For this review, take the finished solid that the model builds, in its own axes (mm). Face numbers are marked on the shaded views. A direction names the side the tool comes from. Round coordinates to 2 decimals unless told otherwise and drop trailing zeros. Write each loop counter-clockwise with the first axis right and the second up, starting at its lowest first coordinate (ties: lowest second). Pieces come first, ordered by that corner, then holes. Notation, with made-up numbers: M 79,-36 L 128,-36 A13 ccw 128,-28 Z; hole C -6.5,32 d1. An arc over 180 degrees is marked long. Write each question's results on one line, items separated by ' | '. Start each with the question number.
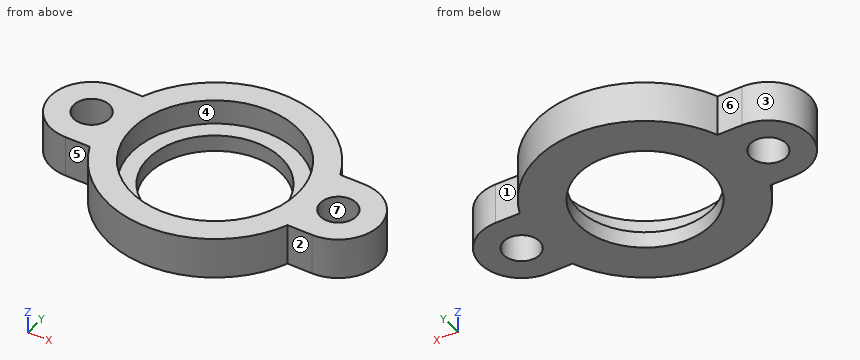
```python
from build123d import *

# Parameters (mm, degrees)
F0_R     = 1.7272
F0_R_2   = 6.4135
F1_DEPTH = 1.5875
F2_R     = 1.7272
F2_R_2   = 8.001
F3_DEPTH = 2.396515


with BuildPart() as f1:
    # F0 (on Top) → F1 (new body)
    with BuildSketch(Plane.XY):
        with BuildLine():
            Line((2.375995, 3.96875), (0, 3.96875))
            ThreePointArc((0, 3.96875), (-3.96875, 0), (0, -3.96875))
            Line((0, -3.96875), (2.375995, -3.96875))
            ThreePointArc((2.375995, -3.96875), (11.96975, -10.38225), (21.563505, -3.96875))
            Line((21.563505, -3.96875), (23.9395, -3.96875))
            ThreePointArc((23.9395, -3.96875), (27.90825, 0), (23.9395, 3.96875))
            Line((23.9395, 3.96875), (21.563505, 3.96875))
            ThreePointArc((21.563505, 3.96875), (11.96975, 10.38225), (2.375995, 3.96875))
        make_face()
        Circle(F0_R, mode=Mode.SUBTRACT)
        with Locations((11.96975, 0)):
            Circle(F0_R_2, mode=Mode.SUBTRACT)
        with Locations((23.9395, 0)):
            Circle(F0_R, mode=Mode.SUBTRACT)
    extrude(amount=F1_DEPTH)

    # F2 (on face) → F3 (join)
    with BuildSketch(Plane.XY.offset(1.5875)):
        with BuildLine():
            Line((23.9395, 3.96875), (21.563505, 3.96875))
            ThreePointArc((21.563505, 3.96875), (11.96975, 10.38225), (2.375995, 3.96875))
            Line((2.375995, 3.96875), (0, 3.96875))
            ThreePointArc((0, 3.96875), (-3.96875, 0), (0, -3.96875))
            Line((0, -3.96875), (2.375995, -3.96875))
            ThreePointArc((2.375995, -3.96875), (11.96975, -10.38225), (21.563505, -3.96875))
            Line((21.563505, -3.96875), (23.9395, -3.96875))
            ThreePointArc((23.9395, -3.96875), (27.90825, 0), (23.9395, 3.96875))
        make_face()
        Circle(F2_R, mode=Mode.SUBTRACT)
        with Locations((11.96975, 0)):
            Circle(F2_R_2, mode=Mode.SUBTRACT)
        with Locations((23.9395, 0)):
            Circle(F2_R, mode=Mode.SUBTRACT)
    extrude(amount=F3_DEPTH)


solid = f1.part
```
Item 1: Mouldability with a two-part tool opening along Y and no side actions: class the marked faces 5, 6 and 7 as pulls with the +Y half, pulls with the -Y half, needs draft (parallel to the pull), parting line crosses it, or undercut.
Item 2: We need section D-D on y = 5.75. State the section outline as (x, z) points, then the cut area to 3 significant figures.
Item 3: For probe 1 along Y at (x, z) = (0, 2.25); probe 2 along X at (y, z) = (-0.75, 3.4); probe 3 along Y at (x, z) = (10.5, 1.55), list the stretches that pass through material, from the lowest coordinate up.
Item 4: We need section B-B on y = 0. State the section outline as (x, z) points, then the cut area to 3 significant figures.
Item 5: We need section A-A on z = 2.9. State the section outline as (x, y) points.
Item 6: For the marked faces 1, 2, 3 and 4, list the 3-axis set-ups (+Z, -Z, +X, -X, +Y, -Y) from which the entire face can be reached by the end or side of a thin tool; tool diameter is ignored.
Item 7: We need section C-C on x = 11. State the section outline as (y, z) points.
Item 8: Insertion check: P1, Ø1, axis at x = 22, z = 3, coming from the -Y side; P2, Ø0.7, axis at x = 23.5, z = 1.5, coming from the -Y side; P3, Ø1, axis at x = 4, z = 2, coming from the +Y side. Each pin has a flat end and moves straight along its axis. Give the tip position at first contact, or say it passes through.
Numbers:
1) face 5: pulls with the -Y half | face 6: pulls with the +Y half | face 7: undercut
2) outline: M 3.33,0 L 9.13,0 L 9.13,1.59 L 6.41,1.59 L 6.41,3.98 L 3.33,3.98 Z; M 14.81,0 L 20.61,0 L 20.61,3.98 L 17.53,3.98 L 17.53,1.59 L 14.81,1.59 Z | area: 33.2 mm^2
3) probe 1: y = -3.97 to -1.73, 1.73 to 3.97 | probe 2: x = -3.9 to -1.56, 1.56 to 4, 19.94 to 22.38, 25.5 to 27.84 | probe 3: y = -10.28 to -6.24, 6.24 to 10.28
4) outline: M -3.97,0 L -1.73,0 L -1.73,3.98 L -3.97,3.98 Z; M 1.73,0 L 5.56,0 L 5.56,1.59 L 3.97,1.59 L 3.97,3.98 L 1.73,3.98 Z; M 18.38,0 L 22.21,0 L 22.21,3.98 L 19.97,3.98 L 19.97,1.59 L 18.38,1.59 Z; M 25.67,0 L 27.91,0 L 27.91,3.98 L 25.67,3.98 Z | area: 40.8 mm^2
5) outline: M 0,-3.97 L 2.38,-3.97 A10.38 ccw 21.56,-3.97 L 23.94,-3.97 A3.97 ccw 23.94,3.97 L 21.56,3.97 A10.38 ccw 2.38,3.97 L 0,3.97 A3.97 ccw Z; hole C 0,0 d3.45; hole C 11.97,0 d16; hole C 23.94,0 d3.45
6) face 1: +Z, -Z, +X, +Y | face 2: +Z, -Z, +X, -Y | face 3: +Z, -Z, -X | face 4: +Z
7) outline: M -10.34,0 L -6.34,0 L -6.34,1.59 L -7.94,1.59 L -7.94,3.98 L -10.34,3.98 Z; M 6.34,0 L 10.34,0 L 10.34,3.98 L 7.94,3.98 L 7.94,1.59 L 6.34,1.59 Z
8) P1: stops at y = -4.12 | P2: stops at y = -3.97 | P3: stops at y = 7.21
